Part model, mm, in its own coordinate system. Face numbers are marked on the shaded views. Round coordinates to 2 decimals unless told otherwise and drop trailing zeros. Loops run counter-clockwise (first coordinate to the right, second up) from the corner with the lowest first, then second, coordinate; pieces in that order, holes last. Notation, with made-up numbers: (56, 31) -> (74, 31) arc R31 ccw to (74, 57) -> close; hole circle Ø8 at (65, -22.75). An arc over 180 degrees is marked (long way). Use a Markdown table: item, result. Add a question column.
Item 1: Cut at A-A, the plane y = 5.5. List the corners of the cut face in (x, z), plus the area to 3 significant figures.
Item 2: Cut at B-B, the plane x = 15. List the corners of the cut face in (y, z).
Item 3: Probe line 1 (X direction, y = 21, z = 379.5); line 2 (Y direction, x = 6, z = 166). List the from-to ranges inside material, lowest first. Write a range as [from, to].
Item 4: Two-plate mould, pull along X, no slides. Class the marked faces 1, 2, 3 and 4: pulls with the +X half, pulls with the -X half, needs draft (parallel to the pull), parting line crosses it, or undercut.
Item 5: Flat gauge pin, fed straight in: pin 1 (12 mm diameter, centred on x = -6.5, z = 182.5, fed in from +Y). Where does the tip first touch, or does it go through?
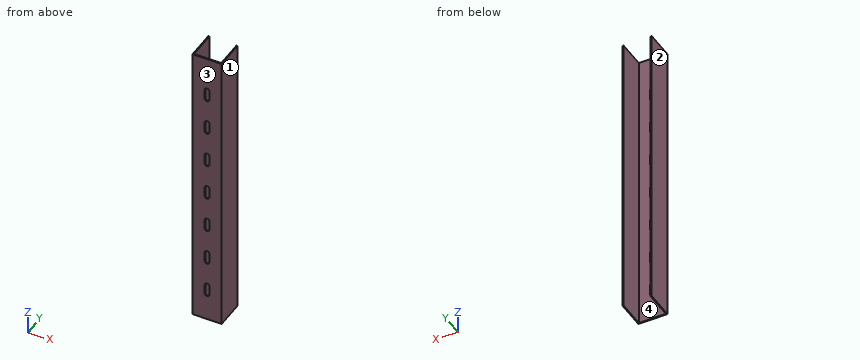
```python
from build123d import *

# Parameters (mm, degrees)
CROQUIS1_W              = 400
CROQUIS1_H              = 40
SALIENTE_EXTRUIR1_DEPTH = 40
CROQUIS2_W              = 37
CROQUIS2_H              = 38.5
CORTAR_EXTRUIR1_DEPTH   = 401
CORTAR_EXTRUIR2_DEPTH   = 2.5
CORTAR_EXTRUIR3_DEPTH   = 2.5
CORTAR_EXTRUIR4_DEPTH   = 2.5
CORTAR_EXTRUIR5_DEPTH   = 2.5
CORTAR_EXTRUIR6_DEPTH   = 2.5
CORTAR_EXTRUIR7_DEPTH   = 2.5
CORTAR_EXTRUIR8_DEPTH   = 41


with BuildPart() as part:
    # Croquis1 → Saliente-Extruir1 (new body)
    with BuildSketch(Plane(origin=(20, 0, 0), x_dir=(0, 0, -1), z_dir=(1, 0, 0))):
        with Locations((-200, 18.5)):
            Rectangle(CROQUIS1_W, CROQUIS1_H)
    extrude(amount=-SALIENTE_EXTRUIR1_DEPTH)

    # Croquis2 → Cortar-Extruir1 (cut, through all)
    with BuildSketch(Plane.XY.offset(400)):
        with Locations((0, 19.25)):
            Rectangle(CROQUIS2_W, CROQUIS2_H)
    extrude(amount=-CORTAR_EXTRUIR1_DEPTH, mode=Mode.SUBTRACT)

    # Croquis3 → Cortar-Extruir2 (cut, through all)
    with BuildSketch(Plane(origin=(0, 0, 0), x_dir=(-1, 0, 0), z_dir=(0, 1, 0))):
        with BuildLine():
            Line((-3.25, 351.5), (-3.25, 338.5))
            ThreePointArc((-3.25, 338.5), (0, 335.25), (3.25, 338.5))
            Line((3.25, 338.5), (3.25, 351.5))
            ThreePointArc((3.25, 351.5), (0, 354.75), (-3.25, 351.5))
        make_face()
    extrude(amount=-CORTAR_EXTRUIR2_DEPTH, mode=Mode.SUBTRACT)

    # Croquis4 → Cortar-Extruir3 (cut, through all)
    with BuildSketch(Plane(origin=(0, 0, 0), x_dir=(-1, 0, 0), z_dir=(0, 1, 0))):
        with BuildLine():
            Line((-3.25, 301.5), (-3.25, 288.5))
            ThreePointArc((-3.25, 288.5), (0, 285.25), (3.25, 288.5))
            Line((3.25, 288.5), (3.25, 301.5))
            ThreePointArc((3.25, 301.5), (0, 304.75), (-3.25, 301.5))
        make_face()
    extrude(amount=-CORTAR_EXTRUIR3_DEPTH, mode=Mode.SUBTRACT)

    # Croquis5 → Cortar-Extruir4 (cut, through all)
    with BuildSketch(Plane(origin=(0, 0, 0), x_dir=(-1, 0, 0), z_dir=(0, 1, 0))):
        with BuildLine():
            Line((-3.25, 251.5), (-3.25, 238.5))
            ThreePointArc((-3.25, 238.5), (0, 235.25), (3.25, 238.5))
            Line((3.25, 238.5), (3.25, 251.5))
            ThreePointArc((3.25, 251.5), (0, 254.75), (-3.25, 251.5))
        make_face()
    extrude(amount=-CORTAR_EXTRUIR4_DEPTH, mode=Mode.SUBTRACT)

    # Croquis6 → Cortar-Extruir5 (cut, through all)
    with BuildSketch(Plane(origin=(0, 0, 0), x_dir=(-1, 0, 0), z_dir=(0, 1, 0))):
        with BuildLine():
            Line((-3.25, 201.5), (-3.25, 188.5))
            ThreePointArc((-3.25, 188.5), (0, 185.25), (3.25, 188.5))
            Line((3.25, 188.5), (3.25, 201.5))
            ThreePointArc((3.25, 201.5), (0, 204.75), (-3.25, 201.5))
        make_face()
    extrude(amount=-CORTAR_EXTRUIR5_DEPTH, mode=Mode.SUBTRACT)

    # Croquis7 → Cortar-Extruir6 (cut, through all)
    with BuildSketch(Plane(origin=(0, 0, 0), x_dir=(-1, 0, 0), z_dir=(0, 1, 0))):
        with BuildLine():
            Line((-3.25, 151.5), (-3.25, 138.5))
            ThreePointArc((-3.25, 138.5), (0, 135.25), (3.25, 138.5))
            Line((3.25, 138.5), (3.25, 151.5))
            ThreePointArc((3.25, 151.5), (0, 154.75), (-3.25, 151.5))
        make_face()
    extrude(amount=-CORTAR_EXTRUIR6_DEPTH, mode=Mode.SUBTRACT)

    # Croquis8 → Cortar-Extruir7 (cut, through all)
    with BuildSketch(Plane(origin=(0, 0, 0), x_dir=(-1, 0, 0), z_dir=(0, 1, 0))):
        with BuildLine():
            Line((-3.25, 101.5), (-3.25, 88.5))
            ThreePointArc((-3.25, 88.5), (0, 85.25), (3.25, 88.5))
            Line((3.25, 88.5), (3.25, 101.5))
            ThreePointArc((3.25, 101.5), (0, 104.75), (-3.25, 101.5))
        make_face()
    extrude(amount=-CORTAR_EXTRUIR7_DEPTH, mode=Mode.SUBTRACT)

    # Croquis9 → Cortar-Extruir8 (cut, through all)
    with BuildSketch(Plane.XZ.offset(1.5)):
        with BuildLine():
            Line((-3.25, 51.5), (-3.25, 38.5))
            ThreePointArc((-3.25, 38.5), (0, 35.25), (3.25, 38.5))
            Line((3.25, 38.5), (3.25, 51.5))
            ThreePointArc((3.25, 51.5), (0, 54.75), (-3.25, 51.5))
        make_face()
    extrude(amount=-CORTAR_EXTRUIR8_DEPTH, mode=Mode.SUBTRACT)


solid = part.part
```
A:
| question | item | result |
|---|---|---|
| 1 | outline | (-20, 0) -> (-18.5, 0) -> (-18.5, 400) -> (-20, 400) -> close; (18.5, 0) -> (20, 0) -> (20, 400) -> (18.5, 400) -> close |
| 1 | area | 1,200 mm^2 |
| 2 | outline | (-1.5, 0) -> (0, 0) -> (0, 400) -> (-1.5, 400) -> close |
| 3 | line 1 | x = [-20, -18.5], [18.5, 20] |
| 3 | line 2 | y = [-1.5, 0] |
| 4 | face 1 | pulls with the +X half |
| 4 | face 2 | pulls with the -X half |
| 4 | face 3 | needs draft |
| 4 | face 4 | undercut |
| 5 | pin 1 | stops at y = 0 |
